Model file for the job. Use its own axes, mm. Face numbers are marked on the shaded views. A direction names the side the tool comes from. Round coordinates to 2 decimals unless told otherwise and drop trailing zeros. Loops run counter-clockwise (first coordinate to the right, second up) from the corner with the lowest first, then second, coordinate; pieces in that order, holes last. Notation, with made-up numbers: M -6,-13.5 L 46,-13.5 A4 ccw 46,-7.5 Z; hole C 24.25,47 d6. An arc over 180 degrees is marked long. Answer in a Markdown table with one row per item.
from build123d import *
from OCP.BRepAlgoAPI import BRepAlgoAPI_Cut
from OCP.TopTools import TopTools_ListOfShape

# Parameters (mm, degrees)
SKETCH1_R           = 6.858
BOSS_EXTRUDE1_DEPTH = 48.26
FILLET1_R           = 0.254
SKETCH2_R           = 2.54
BOSS_EXTRUDE2_DEPTH = 1.27
FILLET2_R           = 0.508


with BuildPart() as part:
    # Sketch1 → Boss-Extrude1 (new body)
    with BuildSketch(Plane.XY):
        with Locations(Location((0, 0, 0), (0, 0, 180))):
            Circle(SKETCH1_R)
    extrude(amount=BOSS_EXTRUDE1_DEPTH)

    # Fillet1
    fillet1_edges = [part.edges().sort_by_distance(p)[0] for p in [
        (6.858, 0, 0),
        (6.858, 0, 48.26),
    ]]
    fillet(fillet1_edges, radius=FILLET1_R)

    # Sketch2 → Boss-Extrude2 (add)
    with BuildSketch(Plane.XY.offset(48.26)):
        Circle(SKETCH2_R)
    extrude(amount=BOSS_EXTRUDE2_DEPTH)

    # Fillet2
    fillet2_edges = [part.edges().sort_by_distance(p)[0] for p in [
        (-2.54, 0, 49.53),
    ]]
    fillet(fillet2_edges, radius=FILLET2_R)


with BuildPart() as dome1_tool:
    # Dome1: read off the stored shape, not the designer's step
    # Dome1 outline → Dome1 (revolve)
    with BuildSketch(Plane.XZ):
        with BuildLine():
            Line((0, 0), (6.604000859, -7e-09))
            ThreePointArc((6.604000859, -7e-09), (3.302024852, 0.019049975), (0, 0.0254))
            Line((0, 0.0254), (0, 0))
        make_face()
    revolve(axis=Axis((0, 0, 0), (0, 0, 1)))


with BuildPart() as part_1:
    add(part.part)

    # Dome1: cut by dome1_tool, with a tolerance
    dome1_stock = TopTools_ListOfShape()
    dome1_stock.Append(part_1.part.wrapped)
    dome1_tools = TopTools_ListOfShape()
    dome1_tools.Append(dome1_tool.part.wrapped)
    dome1_cut = BRepAlgoAPI_Cut()
    dome1_cut.SetArguments(dome1_stock)
    dome1_cut.SetTools(dome1_tools)
    dome1_cut.SetFuzzyValue(0.00001)
    dome1_cut.Build()
    add(Compound.cast(dome1_cut.Shape()).solids(), mode=Mode.REPLACE)


solid = part_1.part
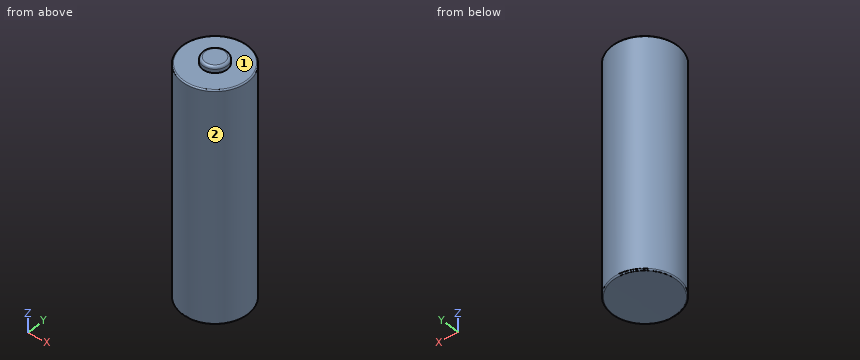
1. Pin check, flat tips, straight feed: pin 1 (2 mm diameter, centred on y = -3.5, z = 10, fed in from -X); pin 2 (4 mm diameter, centred on x = -3, z = 14, fed in from +Y); pin 3 (1 mm diameter, centred on x = -3.5, y = -4, fed in from -Z). Stop position of each tip, or through.
Verdict:
| item | result |
|---|---|
| pin 1 | stops at x = -6.39 |
| pin 2 | stops at y = 6.78 |
| pin 3 | stops at z = 0.01 |
2. Saw through at A-A (z = 42.5). Write the cut outline in (x, y), and give its area (3 significant figures).
Verdict:
| item | result |
|---|---|
| outline | C 0,0 d13.72 |
| area | 148 mm² |
3. Wall check: probe 1 along X at (y, z) = (-0.25, 39.5); probe 2 along Z at (x, y) = (4.25, 2.5); probe 3 along X at (y, z) = (4.75, 46). Give the ranges that are in metal, low to high.
Verdict:
| item | result |
|---|---|
| probe 1 | x = -6.85 to 6.85 |
| probe 2 | z = 0.01 to 48.26 |
| probe 3 | x = -4.95 to 4.95 |
4. Tool access for the marked faces 1 and 2: list every direction of +Z, -Z, +X, -X, +Y, -Y with a clear straight run to the whole face (end or side of a thin tool).
Verdict:
| item | result |
|---|---|
| face 1 | +Z |
| face 2 | +Z, -Z |
